```python
from build123d import *

# Parameters (mm, degrees)
SKETCH1_W           = 16.2
SKETCH1_H           = 108.14
SKETCH1_R           = 0.72
BOSS_EXTRUDE1_DEPTH = 4
FILLET1_R           = 2


with BuildPart() as part:
    # Sketch1 → Boss-Extrude1 (new body)
    with BuildSketch(Plane.XY):
        with Locations((8.1, 54.07)):
            Rectangle(SKETCH1_W, SKETCH1_H)
        with Locations((13.45, 55.21)):
            Circle(SKETCH1_R, mode=Mode.SUBTRACT)
        with Locations((10.2, 48.21)):
            Circle(SKETCH1_R, mode=Mode.SUBTRACT)
        with Locations((13.45, 104.66)):
            Circle(SKETCH1_R, mode=Mode.SUBTRACT)
        with Locations((2.75, 98.16)):
            Circle(SKETCH1_R, mode=Mode.SUBTRACT)
        with Locations((6, 48.21)):
            Circle(SKETCH1_R, mode=Mode.SUBTRACT)
        with Locations((2.75, 27)):
            Circle(SKETCH1_R, mode=Mode.SUBTRACT)
        with Locations((2.75, 87.66)):
            Circle(SKETCH1_R, mode=Mode.SUBTRACT)
        with Locations((2.75, 55.21)):
            Circle(SKETCH1_R, mode=Mode.SUBTRACT)
        with Locations((13.45, 87.66)):
            Circle(SKETCH1_R, mode=Mode.SUBTRACT)
        with Locations((13.45, 98.16)):
            Circle(SKETCH1_R, mode=Mode.SUBTRACT)
        with Locations((13.45, 68.21)):
            Circle(SKETCH1_R, mode=Mode.SUBTRACT)
        with Locations((6, 34)):
            Circle(SKETCH1_R, mode=Mode.SUBTRACT)
        with Locations((2.75, 104.66)):
            Circle(SKETCH1_R, mode=Mode.SUBTRACT)
        with Locations((10.2, 34)):
            Circle(SKETCH1_R, mode=Mode.SUBTRACT)
        with Locations((2.75, 68.21)):
            Circle(SKETCH1_R, mode=Mode.SUBTRACT)
        with Locations((13.45, 27)):
            Circle(SKETCH1_R, mode=Mode.SUBTRACT)
        with Locations((2.85, 10)):
            Circle(SKETCH1_R, mode=Mode.SUBTRACT)
        with Locations((13.35, 10)):
            Circle(SKETCH1_R, mode=Mode.SUBTRACT)
        with Locations((13.35, 4)):
            Circle(SKETCH1_R, mode=Mode.SUBTRACT)
        with Locations((2.85, 4)):
            Circle(SKETCH1_R, mode=Mode.SUBTRACT)
    extrude(amount=BOSS_EXTRUDE1_DEPTH)

    # Fillet1
    fillet1_edges = [part.edges().sort_by_distance(p)[0] for p in [
        (0, 108.14, 2),
        (16.2, 108.14, 2),
    ]]
    fillet(fillet1_edges, radius=FILLET1_R)


solid = part.part
```
Verification items for the finished model (mm, model axes). Round coordinates to 2 decimals unless told otherwise and drop trailing zeros. Write each question's results on one line, items separated by ' | '.
Q1. Go/stop test with a flat-tipped pin: pin 1 Ø1.3 at (x, y) = (2.75, 98.16) entering from -Z. Record where the tip stops, or that it passes through.
Derived:
pin 1: passes through
Q2. Sectioned sample at A-A, the plane z = 2.9. Give the number of separate pieces and of enclosed holes in the cut face, and give its area (3 significant figures).
Derived:
separate pieces: 1 | enclosed holes: 20 | area: 1,720 mm²
Q3. Thickness scan on probe 1 along X at (y, z) = (48.21, 3.15); probe 2 along X at (y, z) = (55.21, 2.85); probe 3 along Y at (x, z) = (6, 0.95). Record the ranges inside material, lowest first.
Derived:
probe 1: x = 0 to 5.28, 6.72 to 9.48, 10.92 to 16.2 | probe 2: x = 0 to 2.03, 3.47 to 12.73, 14.17 to 16.2 | probe 3: y = 0 to 33.28, 34.72 to 47.49, 48.93 to 108.14
